from build123d import *

# Parameters (mm, degrees)
BASPROSKE_W        = 12
BASPROSKE_H        = 8.75
TOOTHCUT_DEPTH     = 18.237314176
TEETHCUTS_COUNT    = 12
TEETHCUTS_ANGLE    = 330
BORSKE_R           = 0.4
BORE_DEPTH         = 50.0000508
SKETCH3_R          = 1.4732
CUT_EXTRUDE1_DEPTH = 17.991923373


with BuildPart() as part:
    # BasProSke → Base-Revolve (revolve)
    with BuildSketch(Plane(origin=(0, 0, 0), x_dir=(1, 0, 0), z_dir=(0, 1, 0)), mode=Mode.PRIVATE) as base_revolve_sk:
        with Locations((6, 4.375)):
            Rectangle(BASPROSKE_W, BASPROSKE_H)
    revolve(base_revolve_sk.sketch.rotate(Axis((-10, 0, 0), (1, 0, 0)), 180), axis=Axis((-10, 0, 0), (1, 0, 0)))

    # TooCutSke → ToothCut (cut, through all)
    with BuildSketch(Plane(origin=(0, 0, 0), x_dir=(0, 0, -1), z_dir=(1, 0, 0))):
        with BuildLine():
            ThreePointArc((0.699286786, 5.895170077), (0, 5.9365), (-0.699286786, 5.895170077))
            ThreePointArc((-0.699286786, 5.895170077), (-1.040581249, 7.393099844), (-2.078649209, 8.525659073))
            ThreePointArc((-2.078649209, 8.525659073), (0, 8.7754), (2.078649209, 8.525659073))
            ThreePointArc((2.078649209, 8.525659073), (1.040581249, 7.393099844), (0.699286786, 5.895170077))
        make_face()
    toothcut = extrude(amount=TOOTHCUT_DEPTH, mode=Mode.SUBTRACT)

    # TeethCuts: ToothCut ×12 about axis
    teethcuts_axis = Axis((-10, 0, 0), (1, 0, 0))
    for i in range(1, TEETHCUTS_COUNT):
        add(toothcut.rotate(teethcuts_axis, i * TEETHCUTS_ANGLE / (TEETHCUTS_COUNT - 1)), mode=Mode.SUBTRACT)

    # BorSke → Bore (cut, symmetric)
    with BuildSketch(Plane(origin=(0, 0, 0), x_dir=(0, 0, -1), z_dir=(1, 0, 0))):
        with Locations(Location((0, 0, 0), (0, 0, 180))):
            Circle(BORSKE_R)
    extrude(amount=BORE_DEPTH, both=True, mode=Mode.SUBTRACT)

    # Sketch3 → Cut-Extrude1 (cut, through all)
    with BuildSketch(Plane(origin=(12, 0, 0), x_dir=(0, 0, -1), z_dir=(1, 0, 0))):
        Circle(SKETCH3_R)
    extrude(amount=-CUT_EXTRUDE1_DEPTH, mode=Mode.SUBTRACT)


solid = part.part
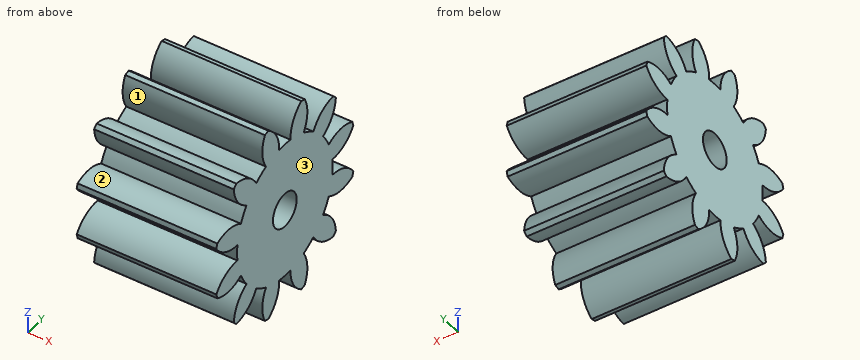
Work out the finished part from the listing and answer in its coordinate system (mm). Face numbers are marked on the shaded views. Give positions to 0.01 mm unless a question says otherwise; leave off trailing zeros. Loops run counter-clockwise (first coordinate to the right, second up) from the corner with the lowest first, then second, coordinate; pieces in that order, holes last. Notation, with made-up numbers: (0.25, 31) -> (19.25, 31) arc R11 cw to (19.25, 39) -> close; hole circle Ø10 at (9, 19). An arc over 180 degrees is marked (long way). Use a Markdown table: item, result. Add a question column.
1. Determine the mould class of the marked faces 1, 2 and 3 for opening direction Z: released by +Z, released by -Z, zero draft, split by the parting line, or undercut.
2. Section A-A on z = 0 is taken. Determine the outline of the cut face in (x, y), and give its area (3 significant figures).
3. Find the intervals of material crossed by probe 1 along Y at (x, z) = (3.75, 0); probe 2 along Y at (x, z) = (2.25, -5); probe 3 along Y at (x, z) = (0.5, -6), in increasing order.
4. Section C-C on z = 4 is taken. Determine the outline of the cut face in (x, y), and give its area (3 significant figures).
5. Flat-ended cylindrical pins translate along their axes: pin 1 Ø5 at (x, z) = (5, 5.5) entering from -Y; pin 2 Ø2 at (x, y) = (1.5, 6) entering from -Z. Find the tip coordinate at first contact, or state that the pin passes through.
6. Section D-D on z = -4.5 is taken. Determine the outline of the cut face in (x, y), and give its area (3 significant figures).
Results below:
| question | item | result |
|---|---|---|
| 1 | face 1 | undercut |
| 1 | face 2 | undercut |
| 1 | face 3 | zero draft |
| 2 | outline | (0, -5.94) -> (12, -5.94) -> (12, -1.47) -> (0, -1.47) -> close; (0, 1.47) -> (12, 1.47) -> (12, 5.94) -> (0, 5.94) -> close |
| 2 | area | 107 mm^2 |
| 3 | probe 1 | y = -5.94 to -1.47, 1.47 to 5.94 |
| 3 | probe 2 | y = -6.1 to -3.7, -3.2 to 3.2, 3.7 to 6.1 |
| 3 | probe 3 | y = -6.34 to -4.8, -2.61 to -0.7, 0.7 to 2.61, 4.8 to 6.34 |
| 4 | outline | (0, -5.38) -> (12, -5.38) -> (12, 5.38) -> (0, 5.38) -> close |
| 4 | area | 129 mm^2 |
| 5 | pin 1 | stops at y = -6.34 |
| 5 | pin 2 | stops at z = -6.34 |
| 6 | outline | (0, -5.82) -> (12, -5.82) -> (12, 5.82) -> (0, 5.82) -> close |
| 6 | area | 140 mm^2 |
